from build123d import *

# Parameters (mm, degrees)
BOSS_EXTRUDE1_DEPTH = 300


with BuildPart() as part:
    # Model → Boss-Extrude1 (new body)
    with BuildSketch(Plane.XY):
        with BuildLine():
            Line((-15, 13), (-15, 4))
            Line((-15, 4), (-13, 4))
            Line((-13, 4), (-13, 8.25))
            Line((-13, 8.25), (-9.664213562, 8.25))
            Line((-9.664213562, 8.25), (-6, 4.585786438))
            Line((-6, 4.585786438), (-6, 0.519615242))
            Line((-6, 0.519615242), (-5.7, 0))
            Line((-5.7, 0), (-5.933012702, -0.403589838))
            ThreePointArc((-5.933012702, -0.403589838), (-6, -0.653589838), (-5.933012702, -0.903589838))
            Line((-5.933012702, -0.903589838), (-5.750976592, -1.218885629))
            Line((-5.750976592, -1.218885629), (-6, -2.5))
            Line((-6, -2.5), (-6, -4.585786438))
            Line((-6, -4.585786438), (-9.664213562, -8.25))
            Line((-9.664213562, -8.25), (-13, -8.25))
            Line((-13, -8.25), (-13, -4))
            Line((-13, -4), (-15, -4))
            Line((-15, -4), (-15, -13))
            ThreePointArc((-15, -13), (-14.414213562, -14.414213562), (-13, -15))
            Line((-13, -15), (-4, -15))
            Line((-4, -15), (-4, -13))
            Line((-4, -13), (-8.25, -13))
            Line((-8.25, -13), (-8.25, -9.664213562))
            Line((-8.25, -9.664213562), (-4.585786438, -6))
            Line((-4.585786438, -6), (-0.519615242, -6))
            Line((-0.519615242, -6), (0, -5.7))
            Line((0, -5.7), (0.403589838, -5.933012702))
            ThreePointArc((0.403589838, -5.933012702), (0.653589838, -6), (0.903589838, -5.933012702))
            Line((0.903589838, -5.933012702), (1.218885629, -5.750976592))
            Line((1.218885629, -5.750976592), (2.5, -6))
            Line((2.5, -6), (4.585786438, -6))
            Line((4.585786438, -6), (8.25, -9.664213562))
            Line((8.25, -9.664213562), (8.25, -13))
            Line((8.25, -13), (4, -13))
            Line((4, -13), (4, -15))
            Line((4, -15), (13, -15))
            ThreePointArc((13, -15), (14.414213562, -14.414213562), (15, -13))
            Line((15, -13), (15, -4))
            Line((15, -4), (13, -4))
            Line((13, -4), (13, -8.25))
            Line((13, -8.25), (9.664213562, -8.25))
            Line((9.664213562, -8.25), (6, -4.585786438))
            Line((6, -4.585786438), (6, -0.519615242))
            Line((6, -0.519615242), (5.7, 0))
            Line((5.7, 0), (5.933012702, 0.403589838))
            ThreePointArc((5.933012702, 0.403589838), (6, 0.653589838), (5.933012702, 0.903589838))
            Line((5.933012702, 0.903589838), (5.750976592, 1.218885629))
            Line((5.750976592, 1.218885629), (6, 2.5))
            Line((6, 2.5), (6, 4.585786438))
            Line((6, 4.585786438), (9.664213562, 8.25))
            Line((9.664213562, 8.25), (13, 8.25))
            Line((13, 8.25), (13, 4))
            Line((13, 4), (15, 4))
            Line((15, 4), (15, 13))
            ThreePointArc((15, 13), (14.414213562, 14.414213562), (13, 15))
            Line((13, 15), (4, 15))
            Line((4, 15), (4, 13))
            Line((4, 13), (8.25, 13))
            Line((8.25, 13), (8.25, 9.664213562))
            Line((8.25, 9.664213562), (4.585786438, 6))
            Line((4.585786438, 6), (0.519615242, 6))
            Line((0.519615242, 6), (0, 5.7))
            Line((0, 5.7), (-0.403589838, 5.933012702))
            ThreePointArc((-0.403589838, 5.933012702), (-0.653589838, 6), (-0.903589838, 5.933012702))
            Line((-0.903589838, 5.933012702), (-1.218885629, 5.750976592))
            Line((-1.218885629, 5.750976592), (-2.5, 6))
            Line((-2.5, 6), (-4.585786438, 6))
            Line((-4.585786438, 6), (-8.25, 9.664213562))
            Line((-8.25, 9.664213562), (-8.25, 13))
            Line((-8.25, 13), (-4, 13))
            Line((-4, 13), (-4, 15))
            Line((-4, 15), (-13, 15))
            ThreePointArc((-13, 15), (-14.414213562, 14.414213562), (-15, 13))
        make_face()
        with BuildLine():
            Line((9.918883282, 12.361530981), (9.539070071, 11.338915743))
            ThreePointArc((9.539070071, 11.338915743), (9.861522369, 9.861522369), (11.338915743, 9.539070071))
            Line((11.338915743, 9.539070071), (12.361530981, 9.918883282))
            ThreePointArc((12.361530981, 9.918883282), (13.043502884, 13.043502884), (9.918883282, 12.361530981))
        make_face(mode=Mode.SUBTRACT)
        with BuildLine():
            Line((12.361530981, -9.918883282), (11.338915743, -9.539070071))
            ThreePointArc((11.338915743, -9.539070071), (9.861522369, -9.861522369), (9.539070071, -11.338915743))
            Line((9.539070071, -11.338915743), (9.918883282, -12.361530981))
            ThreePointArc((9.918883282, -12.361530981), (13.043502884, -13.043502884), (12.361530981, -9.918883282))
        make_face(mode=Mode.SUBTRACT)
        with BuildLine():
            Line((-9.539070071, 11.338915743), (-9.918883282, 12.361530981))
            ThreePointArc((-9.918883282, 12.361530981), (-13.043502884, 13.043502884), (-12.361530981, 9.918883282))
            Line((-12.361530981, 9.918883282), (-11.338915743, 9.539070071))
            ThreePointArc((-11.338915743, 9.539070071), (-9.861522369, 9.861522369), (-9.539070071, 11.338915743))
        make_face(mode=Mode.SUBTRACT)
        with BuildLine():
            Line((-11.338915743, -9.539070071), (-12.361530981, -9.918883282))
            ThreePointArc((-12.361530981, -9.918883282), (-13.043502884, -13.043502884), (-9.918883282, -12.361530981))
            Line((-9.918883282, -12.361530981), (-9.539070071, -11.338915743))
            ThreePointArc((-9.539070071, -11.338915743), (-9.861522369, -9.861522369), (-11.338915743, -9.539070071))
        make_face(mode=Mode.SUBTRACT)
        with BuildLine():
            Line((1.5, 4.335858741), (1.5, 3.5))
            ThreePointArc((1.5, 3.5), (1.374371466, 3.255879964), (1.10270272, 3.21621621))
            ThreePointArc((1.10270272, 3.21621621), (9e-09, 3.4), (-1.102702703, 3.216216216))
            ThreePointArc((-1.102702703, 3.216216216), (-1.374371458, 3.255879959), (-1.5, 3.5))
            Line((-1.5, 3.5), (-1.5, 4.335858741))
            ThreePointArc((-1.5, 4.335858741), (-1.568512625, 4.526682207), (-1.742757301, 4.630346896))
            Line((-1.742757301, 4.630346896), (-2.587190874, 4.794488155))
            ThreePointArc((-2.587190874, 4.794488155), (-2.615679847, 4.79861886), (-2.644433572, 4.8))
            Line((-2.644433572, 4.8), (-4.5, 4.8))
            ThreePointArc((-4.5, 4.8), (-4.712132034, 4.712132034), (-4.8, 4.5))
            Line((-4.8, 4.5), (-4.8, 2.644433572))
            ThreePointArc((-4.8, 2.644433572), (-4.79861886, 2.615679847), (-4.794488155, 2.587190874))
            Line((-4.794488155, 2.587190874), (-4.630346896, 1.742757301))
            ThreePointArc((-4.630346896, 1.742757301), (-4.526682207, 1.568512625), (-4.335858741, 1.5))
            Line((-4.335858741, 1.5), (-3.5, 1.5))
            ThreePointArc((-3.5, 1.5), (-3.255879964, 1.374371466), (-3.21621621, 1.10270272))
            ThreePointArc((-3.21621621, 1.10270272), (-3.4, 9e-09), (-3.216216216, -1.102702703))
            ThreePointArc((-3.216216216, -1.102702703), (-3.255879959, -1.374371458), (-3.5, -1.5))
            Line((-3.5, -1.5), (-4.335858741, -1.5))
            ThreePointArc((-4.335858741, -1.5), (-4.526682207, -1.568512625), (-4.630346896, -1.742757301))
            Line((-4.630346896, -1.742757301), (-4.794488155, -2.587190874))
            ThreePointArc((-4.794488155, -2.587190874), (-4.798618859, -2.615679844), (-4.8, -2.644433568))
            Line((-4.8, -2.644433568), (-4.8, -4.5))
            ThreePointArc((-4.8, -4.5), (-4.712132034, -4.712132034), (-4.5, -4.8))
            Line((-4.5, -4.8), (-2.644433572, -4.8))
            ThreePointArc((-2.644433572, -4.8), (-2.615679847, -4.79861886), (-2.587190874, -4.794488155))
            Line((-2.587190874, -4.794488155), (-1.742757301, -4.630346896))
            ThreePointArc((-1.742757301, -4.630346896), (-1.568512625, -4.526682207), (-1.5, -4.335858741))
            Line((-1.5, -4.335858741), (-1.5, -3.5))
            ThreePointArc((-1.5, -3.5), (-1.374371466, -3.255879964), (-1.10270272, -3.21621621))
            ThreePointArc((-1.10270272, -3.21621621), (-9e-09, -3.4), (1.102702703, -3.216216216))
            ThreePointArc((1.102702703, -3.216216216), (1.374371458, -3.255879959), (1.5, -3.5))
            Line((1.5, -3.5), (1.5, -4.335858741))
            ThreePointArc((1.5, -4.335858741), (1.568512625, -4.526682207), (1.742757301, -4.630346896))
            Line((1.742757301, -4.630346896), (2.587190874, -4.794488155))
            ThreePointArc((2.587190874, -4.794488155), (2.615679847, -4.79861886), (2.644433572, -4.8))
            Line((2.644433572, -4.8), (4.5, -4.8))
            ThreePointArc((4.5, -4.8), (4.712132034, -4.712132034), (4.8, -4.5))
            Line((4.8, -4.5), (4.8, -2.644433572))
            ThreePointArc((4.8, -2.644433572), (4.79861886, -2.615679847), (4.794488155, -2.587190874))
            Line((4.794488155, -2.587190874), (4.630346896, -1.742757301))
            ThreePointArc((4.630346896, -1.742757301), (4.526682207, -1.568512625), (4.335858741, -1.5))
            Line((4.335858741, -1.5), (3.5, -1.5))
            ThreePointArc((3.5, -1.5), (3.255879964, -1.374371466), (3.21621621, -1.10270272))
            ThreePointArc((3.21621621, -1.10270272), (3.4, -9e-09), (3.216216216, 1.102702703))
            ThreePointArc((3.216216216, 1.102702703), (3.255879959, 1.374371458), (3.5, 1.5))
            Line((3.5, 1.5), (4.335858741, 1.5))
            ThreePointArc((4.335858741, 1.5), (4.526682207, 1.568512625), (4.630346896, 1.742757301))
            Line((4.630346896, 1.742757301), (4.794488155, 2.587190874))
            ThreePointArc((4.794488155, 2.587190874), (4.79861886, 2.615679849), (4.8, 2.644433577))
            Line((4.8, 2.644433577), (4.8, 4.5))
            ThreePointArc((4.8, 4.5), (4.712132034, 4.712132034), (4.5, 4.8))
            Line((4.5, 4.8), (2.644433572, 4.8))
            ThreePointArc((2.644433572, 4.8), (2.615679847, 4.79861886), (2.587190874, 4.794488155))
            Line((2.587190874, 4.794488155), (1.742757301, 4.630346896))
            ThreePointArc((1.742757301, 4.630346896), (1.568512625, 4.526682207), (1.5, 4.335858741))
        make_face(mode=Mode.SUBTRACT)
    extrude(amount=BOSS_EXTRUDE1_DEPTH)


solid = part.part
Input: part model. Units: mm. Frame: model coordinates. Round coordinates to 2 decimals unless told otherwise and drop trailing zeros. Answer as a JSON object with one key per item and string values. Group by question number.
(1) Material intervals for probe 1 along X at (y, z) = (11.7, 82); probe 2 along Y at (x, z) = (0, 224), sorted ascending. Write a range as from..to.
(2) Pin query (flat end, axial travel): P1, Ø1.5, axis at x = -1.5, z = 240.5, coming from the -Y side; P2, Ø2.5, axis at x = 11.7, y = -11.7, coming from the +Z side; P3, Ø1, axis at y = 14, z = 90, coming from the +X side; P4, Ø0.6, axis at y = 13.5, z = 171, coming from the -X side. Return the tip coordinate at first contact, or that it passes through.
(3) Cut plane A-A (z = 94.5). Count the separate pieces of the cut face and the enclosed holes in it, then the cut area to 3 significant figures.
Here are the results:
{
 "1": {"probe 1": "x = -15..-13.6, -9.67..-8.25, 8.25..9.67, 13.6..15", "probe 2": "y = -5.7..-3.4, 3.4..5.7"},
 "2": {"P1": "stops at y = -6", "P2": "passes through", "P3": "stops at x = 14.94", "P4": "stops at x = -14.99"},
 "3": {"separate pieces": "1", "enclosed holes": "5", "area": "297 mm^2"}
}
